from build123d import *

# Parameters (mm, degrees)
BOSS_EXTRUDE1_DEPTH = 1.7
SKETCH2_W           = 2.3
SKETCH2_H           = 1.35
CUT_EXTRUDE1_DEPTH  = 0.3
SKETCH3_W           = 0.6
SKETCH3_H           = 0.2
BOSS_EXTRUDE2_DEPTH = 0.25
SKETCH8_W           = 0.6
SKETCH8_H           = 0.2
BOSS_EXTRUDE3_DEPTH = 0.25
SKETCH9_W           = 7.62
SKETCH9_H           = 12.7
BOSS_EXTRUDE4_DEPTH = 2.54
CUT_EXTRUDE2_REACH  = 11.131
SKETCH10_R          = 0.762
SKETCH10_R_2        = 1.5


with BuildPart() as part:
    # Sketch1 → Boss-Extrude1 (new body)
    with BuildSketch(Plane(origin=(0, 0, 0), x_dir=(1, 0, 0), z_dir=(0, 1, 0))):
        Polygon((-1.45, 1.8), (1.45, 1.8), (1.45, -1.8), (-1.05, -1.8), (-1.45, -1.4), align=None)
    extrude(amount=-BOSS_EXTRUDE1_DEPTH)

    # Sketch2 → Cut-Extrude1 (cut)
    with BuildSketch(Plane(origin=(0, 0, 0), x_dir=(1, 0, 0), z_dir=(0, 1, 0))):
        with Locations((0, 0.825)):
            Rectangle(SKETCH2_W, SKETCH2_H)
        Polygon((-1.15, -0.15), (1.15, -0.15), (1.15, -1.5), (-0.925735931, -1.5), (-1.15, -1.275735931), align=None)
    extrude(amount=-CUT_EXTRUDE1_DEPTH, mode=Mode.SUBTRACT)

    # Sketch3 → Boss-Extrude2 (add)
    with BuildSketch(Plane.ZY.offset(1.45)):
        with Locations((-0.9, -1.04)):
            Rectangle(SKETCH3_W, SKETCH3_H)
        with Locations((0.9, -1.04)):
            Rectangle(SKETCH3_W, SKETCH3_H)
    extrude(amount=BOSS_EXTRUDE2_DEPTH)

    # Sketch8 → Boss-Extrude3 (add)
    with BuildSketch(Plane(origin=(1.45, 0, 0), x_dir=(0, 0, -1), z_dir=(1, 0, 0))):
        with Locations((-0.9, -1.1)):
            Rectangle(SKETCH8_W, SKETCH8_H)
        with Locations((0.9, -1.1)):
            Rectangle(SKETCH8_W, SKETCH8_H)
    extrude(amount=BOSS_EXTRUDE3_DEPTH)

    # Sketch9 → Boss-Extrude4 (add)
    with BuildSketch(Plane.XZ.offset(1.7)):
        with Locations((0, 1.55)):
            Rectangle(SKETCH9_W, SKETCH9_H)
    extrude(amount=BOSS_EXTRUDE4_DEPTH)

    # Sketch10 → Cut-Extrude2 (cut, up to next)
    with BuildSketch(Plane(origin=(0, -1.7, 0), x_dir=(1, 0, 0), z_dir=(0, 1, 0)), mode=Mode.PRIVATE) as cut_extrude2_sk1:
        with Locations(Location((0, 3.3, 0), (0, 0, 270))):
            Circle(SKETCH10_R)
    cut_extrude2_tool1 = extrude(cut_extrude2_sk1.sketch, amount=-CUT_EXTRUDE2_REACH, mode=Mode.PRIVATE) & part.part
    # Sketch10 → Cut-Extrude2 (cut, up to next)
    with BuildSketch(Plane(origin=(0, -1.7, 0), x_dir=(1, 0, 0), z_dir=(0, 1, 0)), mode=Mode.PRIVATE) as cut_extrude2_sk2:
        with Locations(Location((2.54, 3.3, 0), (0, 0, 270))):
            Circle(SKETCH10_R)
    cut_extrude2_tool2 = extrude(cut_extrude2_sk2.sketch, amount=-CUT_EXTRUDE2_REACH, mode=Mode.PRIVATE) & part.part
    # Sketch10 → Cut-Extrude2 (cut, up to next)
    with BuildSketch(Plane(origin=(0, -1.7, 0), x_dir=(1, 0, 0), z_dir=(0, 1, 0)), mode=Mode.PRIVATE) as cut_extrude2_sk3:
        with Locations(Location((-2.54, 3.3, 0), (0, 0, 90))):
            Circle(SKETCH10_R)
    cut_extrude2_tool3 = extrude(cut_extrude2_sk3.sketch, amount=-CUT_EXTRUDE2_REACH, mode=Mode.PRIVATE) & part.part
    # Sketch10 → Cut-Extrude2 (cut, up to next)
    with BuildSketch(Plane(origin=(0, -1.7, 0), x_dir=(1, 0, 0), z_dir=(0, 1, 0)), mode=Mode.PRIVATE) as cut_extrude2_sk4:
        with Locations(Location((0, -5.66, 0), (0, 0, 270))):
            Circle(SKETCH10_R_2)
    cut_extrude2_tool4 = extrude(cut_extrude2_sk4.sketch, amount=-CUT_EXTRUDE2_REACH, mode=Mode.PRIVATE) & part.part
    add(cut_extrude2_tool1.solids().sort_by_distance((0, -1.7, -3.3))[0], mode=Mode.SUBTRACT)
    add(cut_extrude2_tool2.solids().sort_by_distance((2.54, -1.7, -3.3))[0], mode=Mode.SUBTRACT)
    add(cut_extrude2_tool3.solids().sort_by_distance((-2.54, -1.7, -3.3))[0], mode=Mode.SUBTRACT)
    add(cut_extrude2_tool4.solids().sort_by_distance((0, -1.7, 5.66))[0], mode=Mode.SUBTRACT)


solid = part.part
Can you work these out from the model? Positions are in its coordinate system, mm. A direction names the side the tool comes from. Give positions to 0.01 mm unless a question says otherwise; leave off trailing zeros. Loops run counter-clockwise (first coordinate to the right, second up) from the corner with the lowest first, then second, coordinate; pieces in that order, holes last. Notation, with made-up numbers: (88, 77) -> (147, 77) arc R26 ccw to (147, 114) -> close; hole circle Ø4 at (7, 18). An arc over 180 degrees is marked (long way). Use one line per item in the form item = value.
1) If we section it at B-B (x = -2.54): Please give me the cut outline in (y, z), plus the area to 3 significant figures.
Answers:
outline = (-4.24, -4.8) -> (-1.7, -4.8) -> (-1.7, -4.06) -> (-4.24, -4.06) -> close; (-4.24, -2.54) -> (-1.7, -2.54) -> (-1.7, 7.9) -> (-4.24, 7.9) -> close
area = 28.4 mm²
2) If we section it at A-A (z = 5.66): Please give me the cut outline in (x, y), plus the area to 3 significant figures.
Answers:
outline = (-3.81, -4.24) -> (-1.5, -4.24) -> (-1.5, -1.7) -> (-3.81, -1.7) -> close; (1.5, -4.24) -> (3.81, -4.24) -> (3.81, -1.7) -> (1.5, -1.7) -> close
area = 11.7 mm²
3) Will these pins go through, and if not, where does the flat tip stop? pin 1 (0.7 mm diameter, centred on x = 0, z = 1, fed in from +Y); pin 2 (3.5 mm diameter, centred on x = 0, z = 5.66, fed in from +Y); pin 3 (0.8 mm diameter, centred on x = -0.5, y = -1, fed in from -Z).
Answers:
pin_1 = -0.3
pin_2 = -1.7
pin_3 = -1.8
4) I need wall thicknesses on line 1 along X through (y, z) = (-3.2, -3.3); line 2 along X through (y, z) = (-2.45, 5.66); line 3 along Z through (x, y) = (-2.54, -2.5). Which ranges of each line are inside material? Lowest first, please.
Answers:
line_1 = -3.81 to -3.3, -1.78 to -0.76, 0.76 to 1.78, 3.3 to 3.81
line_2 = -3.81 to -1.5, 1.5 to 3.81
line_3 = -4.8 to -4.06, -2.54 to 7.9
5) If we section it at D-D (z = -3): Please give me the cut outline in (x, y).
Answers:
outline = (-3.81, -4.24) -> (-3.24, -4.24) -> (-3.24, -1.7) -> (-3.81, -1.7) -> close; (-1.84, -4.24) -> (-0.7, -4.24) -> (-0.7, -1.7) -> (-1.84, -1.7) -> close; (0.7, -4.24) -> (1.84, -4.24) -> (1.84, -1.7) -> (0.7, -1.7) -> close; (3.24, -4.24) -> (3.81, -4.24) -> (3.81, -1.7) -> (3.24, -1.7) -> close
6) For faces 4 (the face through (0, -1, 1.8)), 5 (the face through (0, -3, -4.8)), 6 (the face through (0, -1, -1.8)), 7 (the face through (0, -3, 7.9)), 8 (the face through (0, -0.3, -1)), which set-ups out of +Z, -Z, +X, -X, +Y, -Y let a thin tool reach every point of the face, with its end or its side?
Answers:
face_4 = +Z, +X, -X, +Y
face_5 = -Z, +X, -X, +Y, -Y
face_6 = -Z, +X, -X, +Y
face_7 = +Z, +X, -X, +Y, -Y
face_8 = +Y
7) If we section it at C-C (y = -3.6): Please give me the cut outline in (x, z).
Answers:
outline = (-3.81, -4.8) -> (3.81, -4.8) -> (3.81, 7.9) -> (-3.81, 7.9) -> close; hole circle Ø1.52 at (-2.54, -3.3); hole circle Ø3 at (0, 5.66); hole circle Ø1.52 at (0, -3.3); hole circle Ø1.52 at (2.54, -3.3)
8) We'd pull the mould along X, two halves only. Please class faces 1 (the face through (-3.81, -3, 1)), 2 (the face through (0, -0.3, 1)), 3 (the face through (3.81, -3, 1)): released by +X, released by -X, zero draft, split by the parting line, or undercut.
Answers:
face_1 = released by -X
face_2 = undercut
face_3 = released by +X
